The figure shows three views and two pictorial views of one solid part (mm, origin at its lowest corner). Answer the questions. A direction names the side the tool comes from. Round coordinates to 2 decimals unless told otherwise and drop trailing zeros. Order: outer loops, then holes, each group sorted by start corner. A loop starts at its lowest first (then second) coordinate and runs counter-clockwise, first axis right, second up. Notation, with made-up numbers: (33.5, -3.5) -> (48.5, -3.5) arc R27 ccw to (48.5, 23.5) -> close; hole circle Ø11 at (72.5, -1). An arc over 180 degrees is marked (long way). Return JSON: item names as keys, results as strings. Group by question number.
(1) Each of these flat-tipped pins is pushed along its axis until it touches: pin 1 (2 mm diameter, centred on x = 10, y = 26.5, fed in from +Z); pin 2 (1.5 mm diameter, centred on y = 17, z = 14.5, fed in from -X); pin 3 (5.5 mm diameter, centred on x = 10, y = 41.5, fed in from -Z); pin 4 (8 mm diameter, centred on x = 8, z = 13.5, fed in from +Y). Where does it stop, or does it pass through?
(2) The part is cut by section C-C (z = 18). Determine the outline of the cut face in (x, y).
(3) Which of the six approach directions +Z, -Z, +X, -X, +Y, -Y give full straight-line access (tool end or side, diameter ignored) to the marked faces 1 and 2?
(4) The part is cut by section D-D (y = 8). Determine the outline of the cut face in (x, z), plus the area to 3 significant figures.
(5) The part is cut by section B-B (x = 21). Determine the outline of the cut face in (y, z).
(6) Consider line 1 (Y direction, x = 21, z = 18.35); line 2 (Y direction, x = 10, z = 18.8); line 3 (X direction, y = 51, z = 8.75). Determine where each line is inside the solid, lowest interval first. Write a range as [from, to].
(7) The part is cut by section A-A (y = 26.5). Determine the outline of the cut face in (x, z).
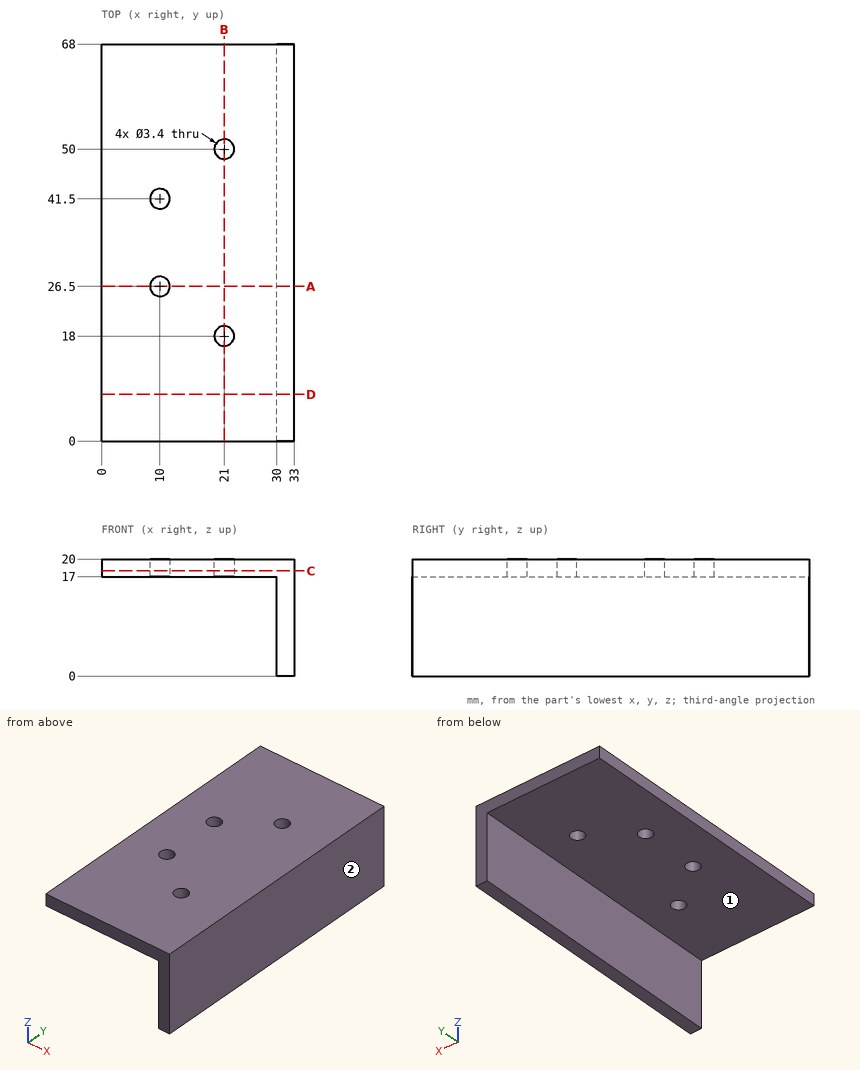
Answer below:
{
 "1": {"pin 1": "passes through", "pin 2": "stops at x = 30", "pin 3": "stops at z = 17", "pin 4": "stops at y = 68"},
 "2": {"outline": "(0, 0) -> (33, 0) -> (33, 68) -> (0, 68) -> close; hole circle Ø3.4 at (10, 26.5); hole circle Ø3.4 at (10, 41.5); hole circle Ø3.4 at (21, 18); hole circle Ø3.4 at (21, 50)"},
 "3": {"face 1": "-Z, -X, +Y, -Y", "face 2": "+Z, -Z, +X, +Y, -Y"},
 "4": {"outline": "(0, 17) -> (30, 17) -> (30, 0) -> (33, 0) -> (33, 20) -> (0, 20) -> close", "area": "150 mm²"},
 "5": {"outline": "(0, 17) -> (16.3, 17) -> (16.3, 20) -> (0, 20) -> close; (19.7, 17) -> (48.3, 17) -> (48.3, 20) -> (19.7, 20) -> close; (51.7, 17) -> (68, 17) -> (68, 20) -> (51.7, 20) -> close"},
 "6": {"line 1": "y = [0, 16.3], [19.7, 48.3], [51.7, 68]", "line 2": "y = [0, 24.8], [28.2, 39.8], [43.2, 68]", "line 3": "x = [30, 33]"},
 "7": {"outline": "(0, 17) -> (8.3, 17) -> (8.3, 20) -> (0, 20) -> close; (11.7, 17) -> (30, 17) -> (30, 0) -> (33, 0) -> (33, 20) -> (11.7, 20) -> close"}
}
